The model under review builds one solid part; all positions refer to its coordinate system, in mm. A direction names the side the tool comes from. Coordinates: 2 decimals unless noted, no trailing zeros. Order: outer loops, then holes, each group sorted by start corner. A loop starts at its lowest first (then second) coordinate and runs counter-clockwise, first axis right, second up. Notation, with made-up numbers: (-27, -7.75) - (23, -7.75) arc R30 cw to (23, 28.25) - close; hole circle Ø8 at (33.25, -38.5). An arc over 180 degrees is marked (long way). Answer in a Markdown table with one row per item.
```python
from build123d import *

# Parameters (mm, degrees)
SKICA2_W                 = 54.6
SKICA2_H                 = 4.2
P_IDAT_VYSUNUT_M2_DEPTH  = 0.4
SKICA3_R                 = 1.75
P_IDAT_VYSUNUT_M3_DEPTH  = 1.5
SKICA5_R                 = 1.9
P_IDAT_VYSUNUT_M5_DEPTH  = 2
ZKOSEN_2_SIZE            = 1.5
SKICA7_W                 = 1
SKICA7_H                 = 5
ODEBRAT_VYSUNUT_M1_DEPTH = 3.5
SKICA8_W                 = 5
SKICA8_H                 = 24.8
P_IDAT_VYSUNUT_M6_DEPTH  = 0.4
SKICA9_R                 = 1.75
P_IDAT_VYSUNUT_M7_DEPTH  = 1.5
SKICA10_R                = 2
P_IDAT_VYSUNUT_M8_DEPTH  = 2
ZKOSEN_3_SIZE            = 1.5
SKICA11_W                = 5
SKICA11_H                = 1
ODEBRAT_VYSUNUT_M2_DEPTH = 3.5


with BuildPart() as part:
    # Skica2 → Přidat vysunutím2 (new body)
    with BuildSketch(Plane.XY):
        Rectangle(SKICA2_W, SKICA2_H)
    extrude(amount=P_IDAT_VYSUNUT_M2_DEPTH)

    # Skica3 → Přidat vysunutím3 (add)
    with BuildSketch(Plane.XY.offset(0.4)):
        with Locations((-20.3, 0)):
            Circle(SKICA3_R)
        with Locations((20.3, 0)):
            Circle(SKICA3_R)
    extrude(amount=P_IDAT_VYSUNUT_M3_DEPTH)

    # Skica5 → Přidat vysunutím5 (add)
    with BuildSketch(Plane.XY.offset(1.9)):
        with Locations((-20.3, 0)):
            Circle(SKICA5_R)
        with Locations((20.3, 0)):
            Circle(SKICA5_R)
    extrude(amount=P_IDAT_VYSUNUT_M5_DEPTH)

    # Zkosení2
    zkosen_2_edges = [part.edges().sort_by_distance(p)[0] for p in [
        (-22.2, 0, 3.9),
        (18.4, 0, 3.9),
    ]]
    chamfer(zkosen_2_edges, length=ZKOSEN_2_SIZE)

    # Skica7 → Odebrat vysunutím1 (cut)
    with BuildSketch(Plane.XY.offset(3.9)):
        with Locations((-20.3, 0)):
            Rectangle(SKICA7_W, SKICA7_H)
        with Locations((20.3, 0)):
            Rectangle(SKICA7_W, SKICA7_H)
    extrude(amount=-ODEBRAT_VYSUNUT_M1_DEPTH, mode=Mode.SUBTRACT)

    # Skica8 → Přidat vysunutím6 (add)
    with BuildSketch(Plane(origin=(0, 0, 0), x_dir=(-1, 0, 0), z_dir=(0, 0, -1))):
        with Locations((0, 14.5)):
            Rectangle(SKICA8_W, SKICA8_H)
    extrude(amount=-P_IDAT_VYSUNUT_M6_DEPTH)

    # Skica9 → Přidat vysunutím7 (add)
    with BuildSketch(Plane.XY.offset(0.4)):
        with Locations((0, 23.910722543)):
            Circle(SKICA9_R)
    extrude(amount=P_IDAT_VYSUNUT_M7_DEPTH)

    # Skica10 → Přidat vysunutím8 (add)
    with BuildSketch(Plane.XY.offset(1.9)):
        with Locations((0, 23.910722543)):
            Circle(SKICA10_R)
    extrude(amount=P_IDAT_VYSUNUT_M8_DEPTH)

    # Zkosení3
    zkosen_3_edges = [part.edges().sort_by_distance(p)[0] for p in [
        (-2, 23.910722543, 3.9),
    ]]
    chamfer(zkosen_3_edges, length=ZKOSEN_3_SIZE)

    # Skica11 → Odebrat vysunutím2 (cut)
    with BuildSketch(Plane.XY.offset(3.9)):
        with Locations((0, 23.910722543)):
            Rectangle(SKICA11_W, SKICA11_H)
    extrude(amount=-ODEBRAT_VYSUNUT_M2_DEPTH, mode=Mode.SUBTRACT)


solid = part.part
```
Item 1: Mouldability with a two-part tool opening along Y and no side actions: class faces 6 (the face through (0.03, 25.66, 1.14)), 7 (the face through (-0.02, 22.67, 3.16)), 8 (the face through (0, 23.411, 2)) as +Y half, -Y half, draft (parallel to the pull), parting line (faces both ways), or undercut.
Check values:
| item | result |
|---|---|
| face 6 | +Y half |
| face 7 | -Y half |
| face 8 | undercut |
Item 2: We need section B-B, the plane x = -12. Write out the cut boundary in (y, z).
Check values:
| item | result |
|---|---|
| outline | (-2.1, 0) - (2.1, 0) - (2.1, 0.4) - (-2.1, 0.4) - close |
Item 3: We need section C-C, the plane y = 4.5. Write out the cut boundary in (x, z), then the cut area to 3 significant figures.
Check values:
| item | result |
|---|---|
| outline | (-2.5, 0) - (2.5, 0) - (2.5, 0.4) - (-2.5, 0.4) - close |
| area | 2.00 mm^2 |
Item 4: We need section A-A, the plane z = 1.2. Write out the cut boundary in (x, y), then the cut area to 3 significant figures.
Check values:
| item | result |
|---|---|
| outline | (-20.8, -1.68) - (-20.8, 1.68) arc R1.75 ccw to start; (-19.8, -1.68) arc R1.75 ccw to (-19.8, 1.68) - close; (-1.68, 23.41) arc R1.75 ccw to (1.68, 23.41) - close; (-1.68, 24.41) - (1.68, 24.41) arc R1.75 ccw to start; (19.8, -1.68) - (19.8, 1.68) arc R1.75 ccw to start; (20.8, -1.68) arc R1.75 ccw to (20.8, 1.68) - close |
| area | 18.5 mm^2 |
Item 5: Tool access review of faces 1 (the face through (22.2, 0, 2.1)), 2 (the face through (-22.2, 0, 2.1)), 3 (the face through (19.8, 0, 2)), 4 (the face through (-0.04, 21.91, 2.15)), 5 (the face through (-0.03, 22.16, 1.14)): name each direction out of +Z, -Z, +X, -X, +Y, -Y from which nothing blocks a thin tool from reaching the whole face with its end or side.
Check values:
| item | result |
|---|---|
| face 1 | +Z, +X |
| face 2 | +Z, -X |
| face 3 | +Z, +Y, -Y |
| face 4 | +Z, -Y |
| face 5 | -Y |
Item 6: To check wall thickness, follow line 1 (X direction, y = -0.25, z = 1.35); line 2 (X direction, y = 4.5, z = 0.2); line 3 (Y direction, x = 0.5, z = 3.2). State the ranges of each line that lie inside material, in increasing order. Write a range as from..to.
Check values:
| item | result |
|---|---|
| line 1 | -22.03..-20.8, -19.8..-18.57, 18.57..19.8, 20.8..22.03 |
| line 2 | -2.5..2.5 |
| line 3 | 22.82..23.41, 24.41..25 |
Item 7: Clearance check with flat-ended pins moving along their axes: pin 1 Ø1.8 at (x, z) = (-1, 2.5) entering from -Y; pin 2 Ø1 at (x, y) = (-19, 3) entering from -Z. State where each tip first meets the part, or that it passes through.
Check values:
| item | result |
|---|---|
| pin 1 | y = 21.91 |
| pin 2 | through |
